from build123d import *

# Parameters (mm, degrees)
BOSS_EXTRUDE1_DEPTH = 4.7625
SKETCH1_3_W         = 6.35
SKETCH1_3_H         = 6.35
BOSS_EXTRUDE2_DEPTH = 27.94
SKETCH2_W           = 19.05
SKETCH2_H           = 6.35
BOSS_EXTRUDE3_DEPTH = 3.175
SKETCH3_W           = 6.35
SKETCH3_H           = 52.959
BOSS_EXTRUDE4_DEPTH = 3.175


with BuildPart() as part:
    # Sketch1 → Boss-Extrude1 (new body)
    with BuildSketch(Plane(origin=(0, 0, 0), x_dir=(1, 0, 0), z_dir=(0, 1, 0))):
        Polygon((-48.895, 3.175), (-48.895, -3.175), (48.895, -3.175), (48.895, 3.175), (-9.525, 3.175), (-9.525, 22.225), (-15.875, 22.225), (-15.875, 3.175), align=None)
    extrude(amount=BOSS_EXTRUDE1_DEPTH)

    # Sketch1_3 → Boss-Extrude2 (add)
    with BuildSketch(Plane(origin=(0, 0, 0), x_dir=(1, 0, 0), z_dir=(0, 1, 0))):
        with Locations((-45.72, 0)):
            Rectangle(SKETCH1_3_W, SKETCH1_3_H)
        with Locations((45.72, 0)):
            Rectangle(SKETCH1_3_W, SKETCH1_3_H)
        with Locations((-12.7, 19.05)):
            Rectangle(SKETCH1_3_W, SKETCH1_3_H)
    extrude(amount=-BOSS_EXTRUDE2_DEPTH)

    # Mirror1: part across plane


with BuildPart() as part_1:
    add(part.part)
    add(part.part.mirror(Plane(origin=(0, 0, 0), x_dir=(0, 0, 1), z_dir=(1, 0, 0))))

    # Sketch2 → Boss-Extrude3 (add)
    with BuildSketch(Plane.XZ.offset(27.94)):
        with Locations((0, -19.05)):
            Rectangle(SKETCH2_W, SKETCH2_H)
        Polygon((-48.895, 3.175), (-48.895, -22.225), (-15.875, -22.225), (-15.875, -15.875), (-42.545, -15.875), (-42.545, 3.175), align=None)
        Polygon((42.545, 3.175), (42.545, -15.875), (15.875, -15.875), (15.875, -22.225), (48.895, -22.225), (48.895, 3.175), align=None)
    extrude(amount=-BOSS_EXTRUDE3_DEPTH)

    # Sketch3 → Boss-Extrude4 (add)
    with BuildSketch(Plane.XZ.offset(27.94)):
        with Locations((-45.72, 29.6545)):
            Rectangle(SKETCH3_W, SKETCH3_H)
    boss_extrude4 = extrude(amount=-BOSS_EXTRUDE4_DEPTH)

    # Mirror2: Boss-Extrude4 across plane
    add(boss_extrude4.mirror(Plane(origin=(0, 0, 0), x_dir=(0, 0, 1), z_dir=(1, 0, 0))))


solid = part_1.part
CAD build for the part. Positions are in the model's coordinates, mm. A direction names the side the tool comes from. Round coordinates to 2 decimals unless told otherwise and drop trailing zeros. Order: outer loops, then holes, each group sorted by start corner. A loop starts at its lowest first (then second) coordinate and runs counter-clockwise, first axis right, second up. Notation, with made-up numbers: M -39,-12.5 L 19,-12.5 A16 cw 19,-1.5 Z; hole C 53.5,0 d1. An arc over 180 degrees is marked long. Use one line per item in the form item = value.
Q1. Saw through at C-C on y = -8. Give the cut face in (x, z) (3 decimals).
Recorded:
outline = M -48.895,-3.175 L -42.545,-3.175 L -42.545,3.175 L -48.895,3.175 Z; M -15.875,-22.225 L -9.525,-22.225 L -9.525,-15.875 L -15.875,-15.875 Z; M 9.525,-22.225 L 15.875,-22.225 L 15.875,-15.875 L 9.525,-15.875 Z; M 42.545,-3.175 L 48.895,-3.175 L 48.895,3.175 L 42.545,3.175 Z
Q2. Saw through at D-D on z = -10. Give the cut face in (x, y) (1 decimal), then the cut area to 3 significant figures.
Recorded:
outline = M -48.9,-27.9 L -42.5,-27.9 L -42.5,-24.8 L -48.9,-24.8 Z; M -15.9,0 L -9.5,0 L -9.5,4.8 L -15.9,4.8 Z; M 9.5,0 L 15.9,0 L 15.9,4.8 L 9.5,4.8 Z; M 42.5,-27.9 L 48.9,-27.9 L 48.9,-24.8 L 42.5,-24.8 Z
area = 101 mm^2
Q3. Which spindle directions (+Z, -Z, +X, -X, +Y, -Y) get a long thin tool onto all of the face, cutting with end or side? Do faces 4 (the flat face through (0, -25, -15.875)), 5 (the flat face through (46, -24.765, 30)), 6 (the flat face through (9.525, -7, -17)), 7 (the flat face through (43, -6, -3.175)). Say none if no direction does.
Recorded:
face_4 = +Z, -Y
face_5 = +Z, +X, -X, +Y
face_6 = -Z, +Y
face_7 = -Z, +X, +Y
Q4. Flat gauge pins, fed straight in: P1, Ø3, axis at x = -2.5, z = -20, coming from the +Y side (3 decimals); P2, Ø6, axis at x = 16.5, z = -8.5, coming from the -Y side; P3, Ø12, axis at x = 21.5, y = -12, coming from the +Z side (3 decimals). Where does each tip first touch, or does it go through?
Recorded:
P1 = -24.765
P2 = 0
P3 = -15.875
Q5. Two-plate mould, pull along X, no slides. Class faces 1 (the flat face through (-48.895, -25, 11)), 2 (the flat face through (-9.525, -7, -17)), 3 (the flat face through (36, -24.765, -17)): +X half, -X half, draft (parallel to the pull), parting line (faces both ways), or undercut.
Recorded:
face_1 = -X half
face_2 = undercut
face_3 = draft
Q6. Probe L1, parallel to X at y = -26, z = 27 (3 decimals); L2, parallel to Z at x = 13.5, y = -27 (3 decimals); L3, parallel to Y at x = -3.5, z = 0. List the from-to ranges inside material, lowest first.
Recorded:
L1 = -48.895 to -42.545, 42.545 to 48.895
L2 = -22.225 to -15.875
L3 = 0 to 4.76
Q7. Saw through at B-B on z = 21. Give the cut face in (x, y) (3 decimals), then the cut area to 3 significant figures.
Recorded:
outline = M -48.895,-27.94 L -42.545,-27.94 L -42.545,-24.765 L -48.895,-24.765 Z; M 42.545,-27.94 L 48.895,-27.94 L 48.895,-24.765 L 42.545,-24.765 Z
area = 40.3 mm^2
Q8. Saw through at A-A on x = 26.5. Give the cut face in (y, z) (1 decimal).
Recorded:
outline = M -27.9,-22.2 L -24.8,-22.2 L -24.8,-15.9 L -27.9,-15.9 Z; M 0,-3.2 L 4.8,-3.2 L 4.8,3.2 L 0,3.2 Z
